from build123d import *

# Parameters (mm, degrees)
SKETCH1_W                = 100
SKETCH1_H                = 130
BOSS_EXTRUDE1_DEPTH      = 15
SKETCH2_W                = 68
SKETCH2_H                = 125
SKETCH2_W_2              = 60
SKETCH2_H_2              = 80
CUT_EXTRUDE1_DEPTH       = 10
SKETCH6_R                = 1.75
CUT_EXTRUDE10_DEPTH      = 15
SKETCH7_W                = 15
SKETCH7_H                = 20
BOSS_EXTRUDE2_DEPTH      = 10
SKETCH8_W                = 15
SKETCH8_H                = 20
BOSS_EXTRUDE3_DEPTH      = 10
CUT_EXTRUDE11_DEPTH      = 40
CUT_EXTRUDE11_DEPTH_BACK = 40
SKETCH9_R                = 2


with BuildPart() as part:
    # Sketch1 → Boss-Extrude1 (new body)
    with BuildSketch(Plane.XY):
        with Locations((150, 65)):
            Rectangle(SKETCH1_W, SKETCH1_H)
        with Locations((50, 65)):
            Rectangle(SKETCH1_W, SKETCH1_H)
    extrude(amount=BOSS_EXTRUDE1_DEPTH)

    # Sketch2 → Cut-Extrude1 (cut)
    with BuildSketch(Plane.XY.offset(15)):
        with Locations((59.584038162, 67.5)):
            Rectangle(SKETCH2_W, SKETCH2_H)
        with Locations((132.534942581, 90)):
            Rectangle(SKETCH2_W_2, SKETCH2_H_2)
    extrude(amount=-CUT_EXTRUDE1_DEPTH, mode=Mode.SUBTRACT)

    # Sketch6 → Cut-Extrude10 (cut)
    with BuildSketch(Plane.XY.offset(15)):
        with Locations((35.063099212, 111.894617683)):
            Circle(SKETCH6_R)
        with Locations((83.399299212, 111.894617683)):
            Circle(SKETCH6_R)
        with Locations((83.399299212, 36.761417683)):
            Circle(SKETCH6_R)
        with Locations((35.063099212, 29.268417683)):
            Circle(SKETCH6_R)
    extrude(amount=-CUT_EXTRUDE10_DEPTH, mode=Mode.SUBTRACT)

    # Sketch7 → Boss-Extrude2 (add)
    with BuildSketch(Plane(origin=(200, 0, 0), x_dir=(0, 0, -1), z_dir=(1, 0, 0))):
        with Locations((-7.5, 120)):
            Rectangle(SKETCH7_W, SKETCH7_H)
    extrude(amount=BOSS_EXTRUDE2_DEPTH)

    # Sketch8 → Boss-Extrude3 (add)
    with BuildSketch(Plane.ZY):
        with Locations((7.5, 10)):
            Rectangle(SKETCH8_W, SKETCH8_H)
    extrude(amount=BOSS_EXTRUDE3_DEPTH)

    # Sketch9 → Cut-Extrude11 (cut, two sides: drawn at the far end of the back side and taken through both)
    with BuildSketch(Plane.XY.offset(15).offset(-CUT_EXTRUDE11_DEPTH_BACK)):
        with Locations((-5, 10)):
            Circle(SKETCH9_R)
        with Locations((205, 120)):
            Circle(SKETCH9_R)
    extrude(amount=CUT_EXTRUDE11_DEPTH + CUT_EXTRUDE11_DEPTH_BACK, mode=Mode.SUBTRACT)


solid = part.part
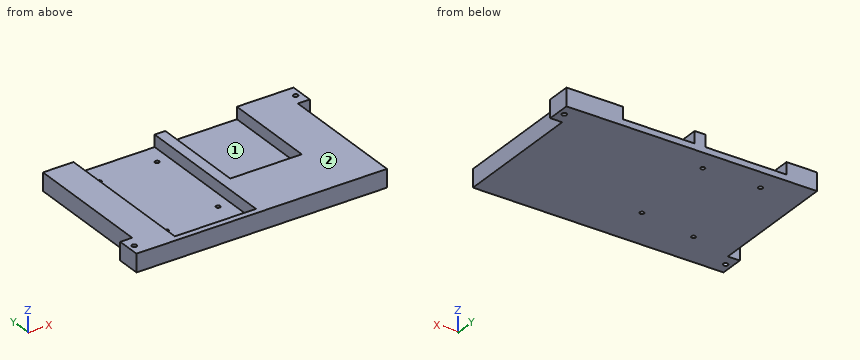
Model file for the job. Use its own axes, mm. Face numbers are marked on the shaded views. A direction names the side the tool comes from. Coordinates: 2 decimals unless noted, no trailing zeros. Loops run counter-clockwise (first coordinate to the right, second up) from the corner with the lowest first, then second, coordinate; pieces in that order, holes last. Notation, with made-up numbers: (5.5, 23) -> (28.5, 23) arc R6 cw to (28.5, 34) -> close; hole circle Ø10 at (73.25, -35). An arc over 180 degrees is marked (long way). Use one line per item in the form item = value. Start each with the question number.
(1) Cut at D-D on x = 124.5. Give the cut face in (y, z), and give its area (3 significant figures).
(2) Cut at C-C on y = 54. Give the cut face in (x, z).
(3) Cut at B-B on x = 77. Give the cut face in (y, z).
(4) Cut at A-A on z = 12.25. Give the cut face in (x, y), and give its area (3 significant figures).
(5) Flat gauge pins, fed straight in: pin 1 (8 mm diameter, centred on y = 55.5, z = 10.5, fed in from +X); pin 2 (4.5 mm diameter, centred on x = 35.06, y = 29.27, fed in from -Z); pin 3 (3 mm diameter, centred on x = 83.4, y = 36.76, fed in from -Z); pin 4 (4.5 mm diameter, centred on y = 94.5, z = 7.5, fed in from -X). Where does each tip first touch, or does it go through?
(6) Tool access for the marked faces 1 and 2: list every direction of +Z, -Z, +X, -X, +Y, -Y with a clear straight run to the whole face (end or side of a thin tool).
(7) Probe probe 1 along X at (y, z) = (103, 6.5); probe 2 along X at (y, z) = (28, 10.25); probe 3 along X at (y, z) = (19, 9.25). List the from-to ranges inside material, lowest first. Write a range as from..to.
Values:
q1.outline = (0, 0) -> (130, 0) -> (130, 5) -> (50, 5) -> (50, 15) -> (0, 15) -> close
q1.area = 1,150 mm2
q2.outline = (0, 0) -> (200, 0) -> (200, 15) -> (162.53, 15) -> (162.53, 5) -> (102.53, 5) -> (102.53, 15) -> (93.58, 15) -> (93.58, 5) -> (25.58, 5) -> (25.58, 15) -> (0, 15) -> close
q3.outline = (0, 0) -> (130, 0) -> (130, 5) -> (5, 5) -> (5, 15) -> (0, 15) -> close
q4.outline = (-10, 0) -> (200, 0) -> (200, 110) -> (210, 110) -> (210, 130) -> (162.53, 130) -> (162.53, 50) -> (102.53, 50) -> (102.53, 130) -> (93.58, 130) -> (93.58, 5) -> (25.58, 5) -> (25.58, 130) -> (0, 130) -> (0, 20) -> (-10, 20) -> close; hole circle Ø4 at (-5, 10); hole circle Ø4 at (205, 120)
q4.area = 13,100 mm2
q5.pin_1 = 200
q5.pin_2 = 0
q5.pin_3 = through
q5.pin_4 = 0
q6.face_1 = +Z, +Y
q6.face_2 = +Z, +X, -X, +Y, -Y
q7.probe_1 = 0..25.58, 93.58..102.53, 162.53..200
q7.probe_2 = 0..25.58, 93.58..200
q7.probe_3 = -10..25.58, 93.58..200
